Geometry: see drawing. Coordinates: mm, zero at the bounding-box minimum. Coordinates: 2 decimals unless noted, no trailing zeros. Order: outer loops, then holes, each group sorted by start corner. A loop starts at its lowest first (then second) coordinate and runs counter-clockwise, first axis right, second up. Notation, with made-up numbers: (-14.5, 38) -> (23.5, 38) arc R31 ccw to (23.5, 75) -> close; hole circle Ø4 at (-8, -22). An arc over 180 degrees is marked (long way). Use one line per item in the form item = value.
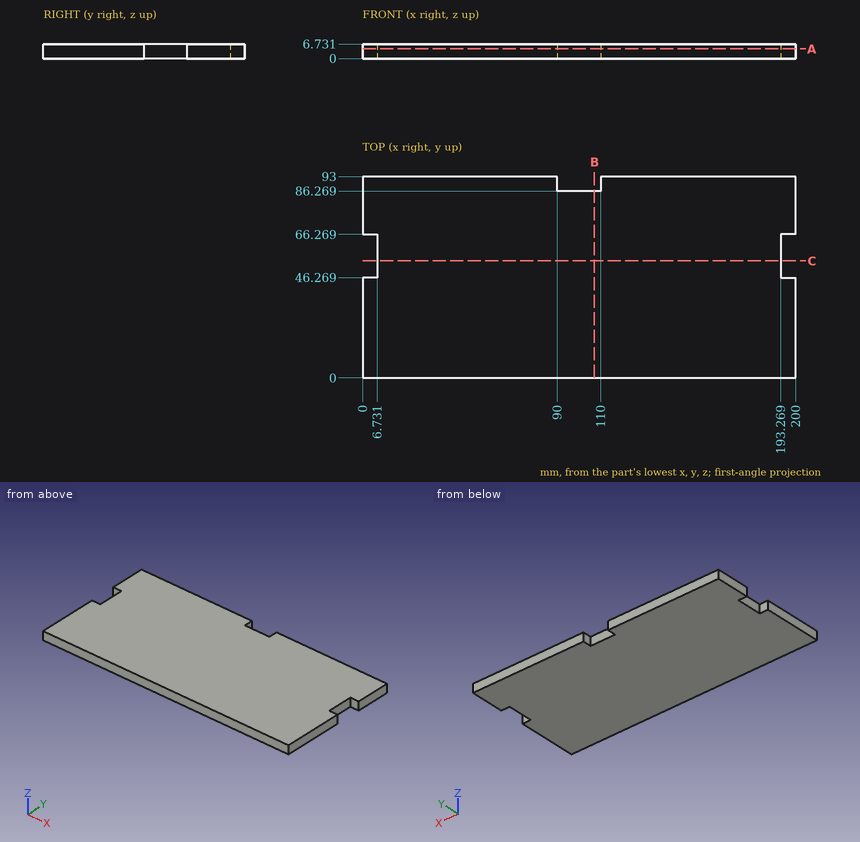
1) Section C-C, the plane y = 54. Output: boundary loops of the cut face in (x, z).
Results found:
outline = (6.73, 0) -> (193.27, 0) -> (193.27, 6.73) -> (6.73, 6.73) -> close
2) Contact query for flat-ended pins moving along their axis: P1, Ø2, axis at y = 59.5, z = 4.5, coming from the +X side; P2, Ø2, axis at x = 100, z = 4, coming from the +Y side. Output: stop coordinate, or through.
Results found:
P1 = 193.27
P2 = 86.27
3) Section B-B, the plane x = 107. Output: boundary loops of the cut face in (y, z), and give its area (3 significant figures).
Results found:
outline = (0, 0) -> (86.27, 0) -> (86.27, 6.73) -> (0, 6.73) -> close
area = 581 mm2
4) Material intervals for probe 1 along X at (y, z) = (48.5, 1.25); probe 2 along Y at (x, z) = (101, 4.5), sorted ascending. Write a range as from..to.
Results found:
probe_1 = 6.73..193.27
probe_2 = 0..86.27
5) Section A-A, the plane z = 4.5. Output: boundary loops of the cut face in (x, y).
Results found:
outline = (0, 0) -> (200, 0) -> (200, 46.27) -> (193.27, 46.27) -> (193.27, 66.27) -> (200, 66.27) -> (200, 93) -> (110, 93) -> (110, 86.27) -> (90, 86.27) -> (90, 93) -> (0, 93) -> (0, 66.27) -> (6.73, 66.27) -> (6.73, 46.27) -> (0, 46.27) -> close
